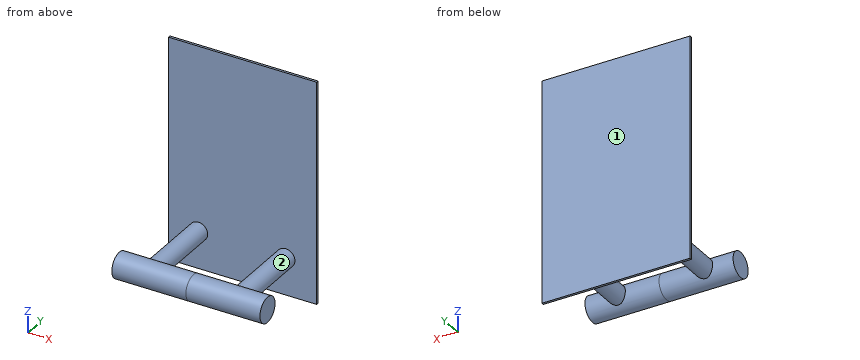
from build123d import *

# Parameters (mm, degrees)
F1_DEPTH      = 1.6002
F2_R          = 6.35
F3_DEPTH      = 50.8
F4_R          = 8.687802
F5_DEPTH      = 50.8
F5_DEPTH_BACK = 50.8


with BuildPart() as f1:
    # F0 (on Front) → F1 (new body)
    with BuildSketch(Plane.XZ):
        Polygon((0, 76.2), (-50.8, 76.2), (-50.8, 0), (-50.8, -76.2), (0, -76.2), (50.8, -76.2), (50.8, 0), (50.8, 76.2), align=None)
    extrude(amount=F1_DEPTH)

    # F2 (on face) → F3 (join)
    with BuildSketch(Plane.XZ.offset(1.6002)):
        with Locations((-30.371312, -50.8)):
            Circle(F2_R)
        with Locations((29.477347, -50.8)):
            Circle(F2_R)
    extrude(amount=F3_DEPTH)

    # F4 (on Right) → F5 (join, two sides)
    with BuildSketch(Plane.YZ) as f5_sk:
        with Locations((-58.367599, -50.84005)):
            Circle(F4_R)
    extrude(amount=F5_DEPTH)
    extrude(f5_sk.sketch, amount=-F5_DEPTH_BACK)


solid = f1.part
Verification items for the finished model (mm, model axes). Face numbers are marked on the shaded views. Coordinates: 2 decimals unless noted, no trailing zeros. Order: outer loops, then holes, each group sorted by start corner. A loop starts at its lowest first (then second) coordinate and runs counter-clockwise, first axis right, second up. Notation, with made-up numbers: M 4.5,9 L 27.5,9 A16 cw 27.5,14 Z; hole C 54,21 d4. An arc over 180 degrees is marked long. Return JSON: item names as keys, results as strings.
1) Release check for a two-part mould opening along X. For the marked faces 1 and 2 record: +X half, -X half, draft (parallel to the pull), parting line (faces both ways), or undercut.
Answer list:
{"face 1": "draft", "face 2": "undercut"}
2) Cross-section at A-A, the plane x = -6. Record the boundary of the cut face in (y, z), and give its area (3 significant figures).
Answer list:
{"outline": "C -58.37,-50.84 d17.38; M -1.6,-76.2 L 0,-76.2 L 0,76.2 L -1.6,76.2 Z", "area": "481 mm2"}
3) Cross-section at B-B, the plane y = -15.5. Record the boundary of the cut face in (x, z), and give its area (3 significant figures).
Answer list:
{"outline": "C -30.37,-50.8 d12.7; C 29.48,-50.8 d12.7", "area": "253 mm2"}
4) Cross-section at C-C, the plane z = 7. Record the boundary of the cut face in (x, y).
Answer list:
{"outline": "M -50.8,-1.6 L 50.8,-1.6 L 50.8,0 L -50.8,0 Z"}
5) Gauge pin test, flat ends, axial feed: pin 1 (1.5 mm diameter, centred on x = -32.5, y = -22, fed in from +Z); pin 2 (3 mm diameter, centred on x = 12, z = 41.5, fed in from -Y). Record the tip position at first contact, or that the pin passes through.
Answer list:
{"pin 1": "z = -44.6", "pin 2": "y = -1.6"}
6) Thickness scan on L1, parallel to Y at x = -15, z = -63; L2, parallel to Y at x = 28.5, z = -44; L3, parallel to X at y = -26, z = -52. Record the ranges inside material, lowest first. Write a range as [from, to].
Answer list:
{"L1": "[-1.6, 0]", "L2": "[-63.72, -53.01], [-1.6, 0]", "L3": "[-36.61, -24.14], [23.24, 35.71]"}
